Input: part model. Units: mm. Frame: model coordinates. A direction names the side the tool comes from. Coordinates: 2 decimals unless noted, no trailing zeros. Loops run counter-clockwise (first coordinate to the right, second up) from the corner with the lowest first, then second, coordinate; pieces in that order, holes last. Notation, with made-up numbers: (60.25, 48.25) -> (84.25, 48.25) arc R27 cw to (84.25, 74.25) -> close; hole circle Ø1 at (-24.5, 60). An arc over 180 degrees is marked (long way). Put each result on its own line as item: value. Start each with the question number.
1) Contact query for flat-ended pins moving along their axis: P1, Ø8, axis at x = 37.24, z = 12.8, coming from the +Y side; P2, Ø11.5, axis at y = -13.5, z = -23.5, coming from the +X side; P3, Ø6, axis at x = 2.5, y = -21.5, coming from the +Z side; P4, Ø3, axis at y = -9.5, z = 28.5, coming from the -X side. Output: stop coordinate, or through.
2) Cut plane C-C (x = 38.5). Return the cut outline in (y, z).
3) Pull-direction query (Z, two-part tool) for faces 4 (the flat face through (40.949, -12.522, -19.293)), 5 (the cylindrical face through (-23.299, -12.522, 43.663)), 6 (the flat face through (-37.238, -13, -26)); classes: pulls with the +Z half, pulls with the -Z half, needs draft (parallel to the pull), parting line crosses it, or undercut.
4) Cut plane B-B (x = -24). Return the cut outline in (y, z), plus the area to 3 significant figures.
5) Set-up query: faces 1 (the flat face through (-22.717, -13, -25)), 2 (the flat face through (-19.079, -12.522, -45.255)), 3 (the flat face through (-51.87, -13, 0)). Return all of +Z, -Z, +X, -X, +Y, -Y with unobstructed straight access to the full face (end or side cutting, diameter ignored); none if empty.
6) Material intervals for L1, parallel to X at y = -9.5, z = -25; L2, parallel to Z at x = -9.5, y = -0.75; L3, parallel to X at y = -3.5, z = 34, sorted ascending.
7) Cut plane D-D (z = -15). Return the cut outline in (x, y).
8) Cut plane A-A (z = -41). Return the cut outline in (x, y), plus the area to 3 significant figures.
from build123d import *

# Parameters (mm, degrees)
F0_R     = 4.4723953016
F0_R_2   = 4.4699433495
F0_R_3   = 4.4865038471
F0_R_4   = 4.4704
F1_DEPTH = 25.4


with BuildPart() as f1:
    # F0 (on Front) → F1 (new body)
    with BuildSketch(Plane.XZ):
        Polygon((-29.8565831035, 42.8078435361), (-29.8565831035, 34.337323159), (-22.7171443403, 30.3440783173), (-15.336762752, 35.2895531338), (-15.336762752, 43.1670817552), (-22.7171443403, 47.285117209), align=None)
        with Locations((-22.7171443403, 39.2283174445)):
            Circle(F0_R, mode=Mode.SUBTRACT)
        Polygon((-22.7171443403, 30.3440783173), (-29.8565831035, 34.337323159), (-37.238035351, 30.3440783173), (-37.238035351, 21.2685223682), (-29.8565831035, 17.1399140715), (-22.7171443403, 19.6934139464), align=None)
        with Locations((-29.8565831035, 25.0187461318)):
            Circle(F0_R_2, mode=Mode.SUBTRACT)
        Polygon((-15.336762752, 43.1670817552), (-15.336762752, 35.2895531338), (-7.5912186876, 30.3440783173), (0, 35.2895531338), (0, 43.0498570204), (-7.3492033407, 47.285117209), align=None)
        with Locations((-7.5912186876, 39.2283174445)):
            Circle(F0_R_3, mode=Mode.SUBTRACT)
        Polygon((-29.8565831035, 17.1399140715), (-37.238035351, 21.2685223682), (-44.7648577392, 17.2623099094), (-44.7648577392, 8.3431052044), (-37.238035351, 4.1331881966), (-29.7259818762, 8.483578451), align=None)
        with Locations((-37.238035351, 12.8027075569)):
            Circle(F0_R_4, mode=Mode.SUBTRACT)
        Polygon((0, 43.0498570204), (0, 35.2895531338), (7.5912186876, 30.3440783173), (15.336762752, 35.2895531338), (15.336762752, 43.1670817552), (7.3492033407, 47.285117209), align=None)
        with Locations((7.5912186876, 39.2283174445)):
            Circle(F0_R_3, mode=Mode.SUBTRACT)
        Polygon((-37.238035351, 4.1331881966), (-44.7648577392, 8.3431052044), (-51.8703386188, 4.5852214098), (-51.8703386188, -4.3693268672), (-44.7648577392, -8.343578319), (-37.2284390032, -4.4903345406), align=None)
        with Locations((-44.7648577392, 0)):
            Circle(F0_R_4, mode=Mode.SUBTRACT)
        Polygon((15.336762752, 43.1670817552), (15.336762752, 35.2895531338), (22.7171443403, 30.3440783173), (29.8565831035, 34.337323159), (29.8565831035, 42.8078435361), (22.7171443403, 47.285117209), align=None)
        with Locations((22.7171443403, 39.2283174445)):
            Circle(F0_R, mode=Mode.SUBTRACT)
        Polygon((-29.7259818762, -8.483578451), (-37.2284390032, -4.4903345406), (-44.7648577392, -8.343578319), (-44.7648577392, -17.2623099094), (-37.238035351, -21.2685223682), (-29.8565831035, -17.1399140715), align=None)
        with Locations((-37.238035351, -12.8027075569)):
            Circle(F0_R_4, mode=Mode.SUBTRACT)
        Polygon((29.8565831035, 34.337323159), (22.7171443403, 30.3440783173), (22.7171443403, 19.6934139464), (29.8565831035, 17.1399140715), (37.238035351, 21.2685223682), (37.238035351, 30.3440783173), align=None)
        with Locations((29.8565831035, 25.0187461318)):
            Circle(F0_R_2, mode=Mode.SUBTRACT)
        Polygon((-22.7171443403, -19.6934139464), (-29.8565831035, -17.1399140715), (-37.238035351, -21.2685223682), (-37.238035351, -30.3440783173), (-29.8565831035, -34.337323159), (-22.7171443403, -30.3440783173), align=None)
        with Locations((-29.8565831035, -25.0187461318)):
            Circle(F0_R_2, mode=Mode.SUBTRACT)
        Polygon((37.238035351, 21.2685223682), (29.8565831035, 17.1399140715), (29.7259818762, 8.483578451), (37.238035351, 4.1331881966), (44.7648577392, 8.3431052044), (44.7648577392, 17.2623099094), align=None)
        with Locations((37.238035351, 12.8027075569)):
            Circle(F0_R_4, mode=Mode.SUBTRACT)
        Polygon((-15.336762752, -35.2895531338), (-22.7171443403, -30.3440783173), (-29.8565831035, -34.337323159), (-29.8565831035, -42.8078435361), (-22.7171443403, -47.285117209), (-15.336762752, -43.1670817552), align=None)
        with Locations((-22.7171443403, -39.2283174445)):
            Circle(F0_R, mode=Mode.SUBTRACT)
        Polygon((0, -35.2895531338), (-7.5912186876, -30.3440783173), (-15.336762752, -35.2895531338), (-15.336762752, -43.1670817552), (-7.3492033407, -47.285117209), (0, -43.0498570204), align=None)
        with Locations((-7.5912186876, -39.2283174445)):
            Circle(F0_R_3, mode=Mode.SUBTRACT)
        Polygon((15.336762752, -35.2895531338), (7.5912186876, -30.3440783173), (0, -35.2895531338), (0, -43.0498570204), (7.3492033407, -47.285117209), (15.336762752, -43.1670817552), align=None)
        with Locations((7.5912186876, -39.2283174445)):
            Circle(F0_R_3, mode=Mode.SUBTRACT)
        Polygon((44.7648577392, 8.3431052044), (37.238035351, 4.1331881966), (37.2284390032, -4.4903345406), (44.7648577392, -8.343578319), (51.8703386188, -4.3693268672), (51.8703386188, 4.5852214098), align=None)
        with Locations((44.7648577392, 0)):
            Circle(F0_R_4, mode=Mode.SUBTRACT)
        Polygon((37.2284390032, -4.4903345406), (29.7259818762, -8.483578451), (29.8565831035, -17.1399140715), (37.238035351, -21.2685223682), (44.7648577392, -17.2623099094), (44.7648577392, -8.343578319), align=None)
        with Locations((37.238035351, -12.8027075569)):
            Circle(F0_R_4, mode=Mode.SUBTRACT)
        Polygon((29.8565831035, -17.1399140715), (22.7171443403, -19.6934139464), (22.7171443403, -30.3440783173), (29.8565831035, -34.337323159), (37.238035351, -30.3440783173), (37.238035351, -21.2685223682), align=None)
        with Locations((29.8565831035, -25.0187461318)):
            Circle(F0_R_2, mode=Mode.SUBTRACT)
        Polygon((22.7171443403, -30.3440783173), (15.336762752, -35.2895531338), (15.336762752, -43.1670817552), (22.7171443403, -47.285117209), (29.8565831035, -42.8078435361), (29.8565831035, -34.337323159), align=None)
        with Locations((22.7171443403, -39.2283174445)):
            Circle(F0_R, mode=Mode.SUBTRACT)
    extrude(amount=F1_DEPTH)


solid = f1.part
Results found:
1. P1: passes through
1. P2: stops at x = 43.85
1. P3: stops at z = 46.22
1. P4: stops at x = -37.24
2. outline: (-25.4, -20.6) -> (0, -20.6) -> (0, -17.09) -> (-25.4, -17.09) -> close; (-25.4, -8.51) -> (0, -8.51) -> (0, 8.51) -> (-25.4, 8.51) -> close; (-25.4, 17.09) -> (0, 17.09) -> (0, 20.6) -> (-25.4, 20.6) -> close
3. face 4: pulls with the -Z half
3. face 5: undercut
3. face 6: needs draft
4. outline: (-25.4, -46.48) -> (0, -46.48) -> (0, -43.51) -> (-25.4, -43.51) -> close; (-25.4, -34.94) -> (0, -34.94) -> (0, -19.23) -> (-25.4, -19.23) -> close; (-25.4, 19.23) -> (0, 19.23) -> (0, 34.94) -> (-25.4, 34.94) -> close; (-25.4, 43.51) -> (0, 43.51) -> (0, 46.48) -> (-25.4, 46.48) -> close
4. area: 949 mm2
5. face 1: +Y, -Y
5. face 2: -Z, +Y, -Y
5. face 3: +Z, -Z, -X, +Y, -Y
6. L1: x = -37.24 to -34.33, -25.39 to -22.72, 22.72 to 25.39, 34.33 to 37.24
6. L2: z = -46.18 to -43.29, -35.17 to -31.56, 31.56 to 35.17, 43.29 to 46.18
6. L3: x = -30.48 to -17.26, -13.32 to -1.98, 1.98 to 13.32, 17.26 to 30.48
7. outline: (-44.76, -25.4) -> (-41.13, -25.4) -> (-41.13, 0) -> (-44.76, 0) -> close; (-33.34, -25.4) -> (-29.82, -25.4) -> (-29.82, 0) -> (-33.34, 0) -> close; (29.82, -25.4) -> (33.34, -25.4) -> (33.34, 0) -> (29.82, 0) -> close; (41.13, -25.4) -> (44.76, -25.4) -> (44.76, 0) -> (41.13, 0) -> close
8. outline: (-29.86, -25.4) -> (-26.82, -25.4) -> (-26.82, 0) -> (-29.86, 0) -> close; (-18.61, -25.4) -> (-11.71, -25.4) -> (-11.71, 0) -> (-18.61, 0) -> close; (-3.47, -25.4) -> (3.47, -25.4) -> (3.47, 0) -> (-3.47, 0) -> close; (11.71, -25.4) -> (18.61, -25.4) -> (18.61, 0) -> (11.71, 0) -> close; (26.82, -25.4) -> (29.86, -25.4) -> (29.86, 0) -> (26.82, 0) -> close
8. area: 681 mm2
